Geometry check sheet. Reference: drawing and pictorial views, mm from the part's lowest x, y, z. Give positions to 0.01 mm unless a question says otherwise; leave off trailing zeros. Loops run counter-clockwise (first coordinate to the right, second up) from the corner with the lowest first, then second, coordinate; pieces in that order, holes last. Notation, with made-up numbers: (2.5, 43) -> (47.5, 43) arc R23 ccw to (47.5, 60) -> close; hole circle Ø11 at (38.5, -33.75). An arc over 180 degrees is marked (long way). Answer in a Markdown table with one row per item. Add a question column.
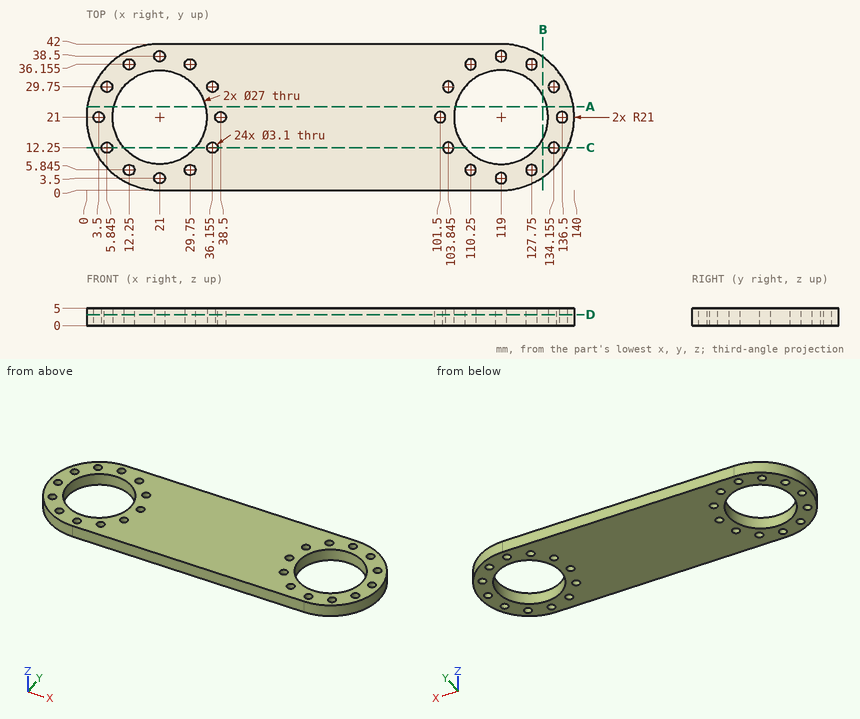
1. Sectioned sample at A-A (y = 24). Enter the section's corners in (x, z) (1 decimal).
2. Sectioned sample at D-D (z = 3.2). Count the separate pieces of the cut face and the enclosed holes in it.
3. Gauge pin test, flat end, axial feed: pin 1 Ø3 at (x, y) = (12.25, 36.16) entering from +Z. Record the tip position at first contact, or that the pin passes through.
4. Sectioned sample at C-C (y = 12.25). Enter the section's corners in (x, z) (1 decimal).
5. Material ranges on L1, parallel to Y at x = 21, z = 4.05; L2, parallel to Y at x = 30, z = 3 (1 decimal); L3, parallel to X at y = 25, z = 0.6 (1 decimal), recorded low to high. Write a range as from..to.
6. Sectioned sample at B-B (x = 131). Enter the section's corners in (y, z) (1 decimal).
Response:
| question | item | result |
|---|---|---|
| 1 | outline | (0.2, 0) -> (7.8, 0) -> (7.8, 5) -> (0.2, 5) -> close; (34.2, 0) -> (105.8, 0) -> (105.8, 5) -> (34.2, 5) -> close; (132.2, 0) -> (139.8, 0) -> (139.8, 5) -> (132.2, 5) -> close |
| 2 | separate pieces | 1 |
| 2 | enclosed holes | 26 |
| 3 | pin 1 | passes through |
| 4 | outline | (1.9, 0) -> (4.3, 0) -> (4.3, 5) -> (1.9, 5) -> close; (7.4, 0) -> (10.7, 0) -> (10.7, 5) -> (7.4, 5) -> close; (31.3, 0) -> (34.6, 0) -> (34.6, 5) -> (31.3, 5) -> close; (37.7, 0) -> (102.3, 0) -> (102.3, 5) -> (37.7, 5) -> close; (105.4, 0) -> (108.7, 0) -> (108.7, 5) -> (105.4, 5) -> close; (129.3, 0) -> (132.6, 0) -> (132.6, 5) -> (129.3, 5) -> close; (135.7, 0) -> (138.1, 0) -> (138.1, 5) -> (135.7, 5) -> close |
| 5 | L1 | y = 0..1.95, 5.05..7.5, 34.5..36.95, 40.05..42 |
| 5 | L2 | y = 0..4.3, 7.4..10.9, 31.1..34.6, 37.7..42 |
| 5 | L3 | x = 0.4..8.1, 33.9..106.1, 131.9..139.6 |
| 6 | outline | (3.8, 0) -> (14.8, 0) -> (14.8, 5) -> (3.8, 5) -> close; (27.2, 0) -> (38.2, 0) -> (38.2, 5) -> (27.2, 5) -> close |
